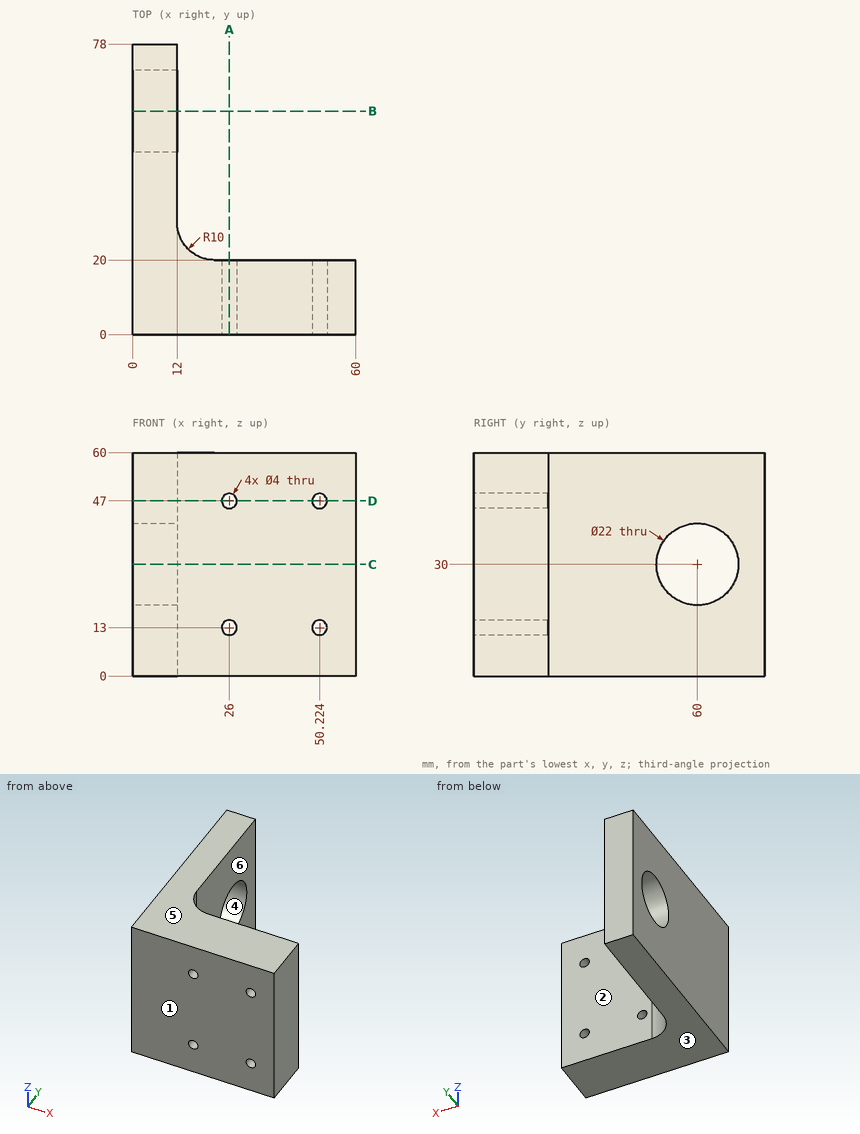
Part print with two shaded views. Sizes in mm from the minimum x, y, z corner. A direction names the side the tool comes from. Round coordinates to 2 decimals unless told otherwise and drop trailing zeros. Order: outer loops, then holes, each group sorted by start corner. A loop starts at its lowest first (then second) coordinate and runs counter-clockwise, first axis right, second up. Notation, with made-up numbers: M -20.5,20 L -15.5,20 A15 cw -15.5,33 Z; hole C 80,-17 d11. An arc over 180 degrees is marked long. Use CSV: the item, a comma, the result in double quotes.
Item 1: Saw through at C-C (z = 30). List the corners of the cut face in (x, y).
Worked answers:
outline,"M 0,0 L 60,0 L 60,20 L 22,20 A10 cw 12,30 L 12,49 L 0,49 Z; M 0,71 L 12,71 L 12,78 L 0,78 Z"
Item 2: Probe probe 1 along X at (y, z) = (8, 47); probe 2 along Y at (x, z) = (8.75, 30); probe 3 along Z at (x, y) = (26, 4). List the from-to ranges inside material, lowest first.
Worked answers:
probe 1,"0 to 24, 28 to 48.22, 52.22 to 60"
probe 2,"0 to 49, 71 to 78"
probe 3,"0 to 11, 15 to 45, 49 to 60"
Item 3: Pull direction Y, two halves, no side cores. Call the marked faces 1, 2, 3 and 4: released by +Y, released by -Y, zero draft, split by the parting line, or undercut.
Worked answers:
face 1,"released by -Y"
face 2,"released by +Y"
face 3,"zero draft"
face 4,"undercut"
Item 4: Saw through at B-B (y = 60). List the corners of the cut face in (x, z), plus the area to 3 significant figures.
Worked answers:
outline,"M 0,0 L 12,0 L 12,19 L 0,19 Z; M 0,41 L 12,41 L 12,60 L 0,60 Z"
area,"456 mm²"
Item 5: Pin check, flat tips, straight feed: pin 1 (1 mm diameter, centred on y = 23, z = 29.5, fed in from +X); pin 2 (19 mm diameter, centred on x = 45.5, z = 18.5, fed in from +Y); pin 3 (6 mm diameter, centred on y = 59, z = 53.5, fed in from +X); pin 4 (3.5 mm diameter, centred on x = 50.22, z = 47, fed in from +Y). Stop position of each tip, or through.
Worked answers:
pin 1,"x = 15.39"
pin 2,"y = 20"
pin 3,"x = 12"
pin 4,"through"
Item 6: Saw through at D-D (z = 47). List the corners of the cut face in (x, y).
Worked answers:
outline,"M 0,0 L 24,0 L 24,20 L 22,20 A10 cw 12,30 L 12,78 L 0,78 Z; M 28,0 L 48.22,0 L 48.22,20 L 28,20 Z; M 52.22,0 L 60,0 L 60,20 L 52.22,20 Z"
Item 7: Saw through at A-A (x = 26). List the corners of the cut face in (y, z), plus the area to 3 significant figures.
Worked answers:
outline,"M 0,0 L 20,0 L 20,11 L 0,11 Z; M 0,15 L 20,15 L 20,45 L 0,45 Z; M 0,49 L 20,49 L 20,60 L 0,60 Z"
area,"1,040 mm²"
Item 8: Which spindle directions (+Z, -Z, +X, -X, +Y, -Y) get a long thin tool onto all of the face, cutting with end or side? Do the marked faces 5 and 6. Say none if no direction does.
Worked answers:
face 5,"+Z, +X, -X, +Y, -Y"
face 6,"+Z, -Z, +X, +Y"
